Can you work these out from the model? Positions are in its coordinate system, mm. Give positions to 0.01 mm unless a question says otherwise; leave off trailing zeros. Loops run counter-clockwise (first coordinate to the right, second up) from the corner with the lowest first, then second, coordinate; pieces in that order, holes last. Notation, with made-up numbers: (27, 77.5) - (83, 77.5) arc R20 ccw to (83, 101.5) - close; hole circle Ø5 at (-25, 56.25). An arc over 180 degrees is marked (long way). Use a Markdown table: item, result. Add a question column.
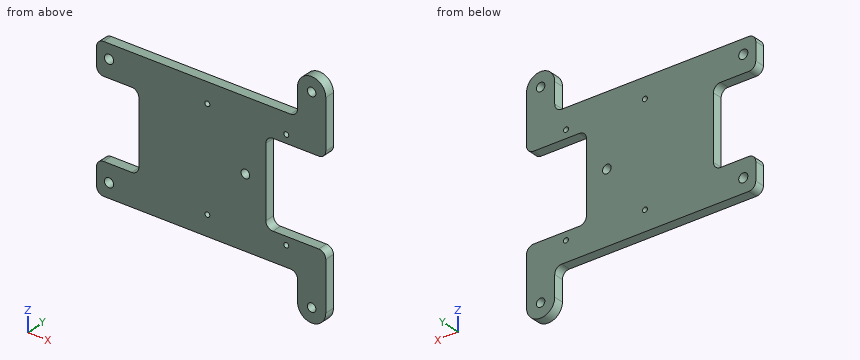
```python
from build123d import *

# Parameters (mm, degrees)
CROQUIS2_R              = 3
CROQUIS2_R_2            = 3.25
SALIENTE_EXTRUIR1_DEPTH = 7
CORTAR_EXTRUIR3_DEPTH   = 7
CROQUIS4_W              = 60
CROQUIS4_H              = 55
CORTAR_EXTRUIR4_DEPTH   = 7
REDONDEO1_R             = 5
CORTAR_EXTRUIR5_DEPTH   = 10
REDONDEO2_R             = 5


with BuildPart() as part:
    # Croquis2 → Saliente-Extruir1 (new body)
    with BuildSketch(Plane(origin=(0, 8, 0), x_dir=(1, 0, 0), z_dir=(0, 1, 0))):
        with BuildLine():
            Line((162.6, -69.675), (162.6, 69.675))
            ThreePointArc((162.6, 69.675), (152.6, 79.675), (142.6, 69.675))
            Line((142.6, 69.675), (142.6, 50.075))
            Line((142.6, 50.075), (8.85, 50.075))
            Line((8.85, 50.075), (0, 50.075))
            Line((0, 50.075), (0, -50.075))
            Line((0, -50.075), (8.85, -50.075))
            Line((8.85, -50.075), (142.6, -50.075))
            Line((142.6, -50.075), (142.6, -69.675))
            ThreePointArc((142.6, -69.675), (152.6, -79.675), (162.6, -69.675))
        make_face()
        with Locations(Location((152.6, -69.675, 0), (0, 0, 90))):
            Circle(CROQUIS2_R, mode=Mode.SUBTRACT)
        with Locations(Location((8.85, -39.925, 0), (0, 0, 90))):
            Circle(CROQUIS2_R_2, mode=Mode.SUBTRACT)
        with Locations(Location((8.85, 39.925, 0), (0, 0, 90))):
            Circle(CROQUIS2_R_2, mode=Mode.SUBTRACT)
        with Locations(Location((152.6, 69.675, 0), (0, 0, 90))):
            Circle(CROQUIS2_R, mode=Mode.SUBTRACT)
    extrude(amount=SALIENTE_EXTRUIR1_DEPTH)

    # Croquis3 → Cortar-Extruir3 (cut)
    with BuildSketch(Plane(origin=(0, 15, 0), x_dir=(1, 0, 0), z_dir=(0, 1, 0))):
        with BuildLine():
            ThreePointArc((134.6, 34.049999999), (136.35, 35.799999999), (134.6, 37.549999999))
            ThreePointArc((134.6, 37.549999999), (132.85, 35.799999999), (134.6, 34.049999999))
        make_face()
        with BuildLine():
            ThreePointArc((78.6, 34.049999999), (80.35, 35.799999999), (78.6, 37.549999999))
            ThreePointArc((78.6, 37.549999999), (76.85, 35.799999999), (78.6, 34.049999999))
        make_face()
        with BuildLine():
            ThreePointArc((134.6, -34.050000001), (132.85, -35.800000001), (134.6, -37.550000001))
            ThreePointArc((134.6, -37.550000001), (136.35, -35.800000001), (134.6, -34.050000001))
        make_face()
        with BuildLine():
            ThreePointArc((78.6, -37.550000001), (80.35, -35.800000001), (78.6, -34.050000001))
            ThreePointArc((78.6, -34.050000001), (76.85, -35.800000001), (78.6, -37.550000001))
        make_face()
        with BuildLine():
            ThreePointArc((105.6, -3.052700001), (108.6527, -1e-09), (105.6, 3.052699999))
            ThreePointArc((105.6, 3.052699999), (102.5473, -1e-09), (105.6, -3.052700001))
        make_face()
    extrude(amount=-CORTAR_EXTRUIR3_DEPTH, mode=Mode.SUBTRACT)

    # Croquis4 → Cortar-Extruir4 (cut)
    with BuildSketch(Plane(origin=(0, 15, 0), x_dir=(1, 0, 0), z_dir=(0, 1, 0))):
        Rectangle(CROQUIS4_W, CROQUIS4_H)
    extrude(amount=-CORTAR_EXTRUIR4_DEPTH, mode=Mode.SUBTRACT)

    # Redondeo1
    redondeo1_edges = [part.edges().sort_by_distance(p)[0] for p in [
        (142.6, 11.5, 50.075),
        (0, 11.5, 50.075),
        (0, 11.5, -50.075),
        (142.6, 11.5, -50.075),
        (0, 11.5, -27.5),
        (0, 11.5, 27.5),
        (30, 11.5, 27.5),
        (30, 11.5, -27.5),
    ]]
    fillet(redondeo1_edges, radius=REDONDEO1_R)

    # Croquis5 → Cortar-Extruir5 (cut)
    with BuildSketch(Plane(origin=(0, 15, 0), x_dir=(1, 0, 0), z_dir=(0, 1, 0))):
        with BuildLine():
            Line((125.1, -30), (205.1, -30))
            Line((205.1, -30), (205.1, 30))
            Line((205.1, 30), (125.1, 30))
            ThreePointArc((125.1, 30), (121.564466094, 28.535533906), (120.1, 25))
            Line((120.1, 25), (120.1, -25))
            ThreePointArc((120.1, -25), (121.564466094, -28.535533906), (125.1, -30))
        make_face()
    extrude(amount=-CORTAR_EXTRUIR5_DEPTH, mode=Mode.SUBTRACT)

    # Redondeo2
    redondeo2_edges = [part.edges().sort_by_distance(p)[0] for p in [
        (162.6, 11.5, -30),
        (162.6, 11.5, 30),
    ]]
    fillet(redondeo2_edges, radius=REDONDEO2_R)


solid = part.part
```
1. Suppose I cut it at D-D (y = 10). State how many separate pieces and enclosed holes the cut face has, and give its area (3 significant figures).
2. Suppose I cut it at A-A (x = 8.85). List the corners of the cut face in (y, z) for me (3 decimals).
3. Suppose I cut it at B-B (z = 0). List the corners of the cut face in (x, y) for me.
4. Please list where these lines run through material, in increasing order: line 1 along X through (y, z) = (11.75, -35.8); line 2 along Z through (x, y) = (78.6, 13.5) (3 decimals); line 3 along Z through (x, y) = (134.6, 12.75) (3 decimals). Write a range as [from, to].
5. Will these pins go through, and if not, where does the flat tip stop? P1, Ø4, axis at x = 48, y = 14, coming from the -Z side (3 decimals); P2, Ø5.5, axis at x = 105.6, z = 0, coming from the -Y side; P3, Ø3.5, axis at x = 95.5, y = 13, coming from the +Z side (3 decimals); P4, Ø2, axis at y = 10.5, z = 10.5, coming from the +X side.
6. Suppose I cut it at C-C (z = -41). List the corners of the cut face in (x, y) for me, and give its area (3 significant figures).
Results below:
| question | item | result |
|---|---|---|
| 1 | separate pieces | 1 |
| 1 | enclosed holes | 9 |
| 1 | area | 13,000 mm² |
| 2 | outline | (8, -50.075) - (15, -50.075) - (15, -43.175) - (8, -43.175) - close; (8, -36.675) - (15, -36.675) - (15, -27.5) - (8, -27.5) - close; (8, 27.5) - (15, 27.5) - (15, 36.675) - (8, 36.675) - close; (8, 43.175) - (15, 43.175) - (15, 50.075) - (8, 50.075) - close |
| 3 | outline | (30, 8) - (102.55, 8) - (102.55, 15) - (30, 15) - close; (108.65, 8) - (120.1, 8) - (120.1, 15) - (108.65, 15) - close |
| 4 | line 1 | [0, 76.85], [80.35, 132.85], [136.35, 162.6] |
| 4 | line 2 | [-50.075, -37.55], [-34.05, 34.05], [37.55, 50.075] |
| 4 | line 3 | [-50.075, -37.55], [-34.05, -30], [30, 34.05], [37.55, 50.075] |
| 5 | P1 | z = -50.075 |
| 5 | P2 | through |
| 5 | P3 | z = 50.075 |
| 5 | P4 | x = 120.1 |
| 6 | outline | (0, 8) - (5.78, 8) - (5.78, 15) - (0, 15) - close; (11.92, 8) - (162.6, 8) - (162.6, 15) - (11.92, 15) - close |
| 6 | area | 1,100 mm² |
